Geometry check sheet. Reference: drawing and pictorial views, mm from the part's lowest x, y, z. A direction names the side the tool comes from. Round coordinates to 2 decimals unless told otherwise and drop trailing zeros. Loops run counter-clockwise (first coordinate to the right, second up) from the corner with the lowest first, then second, coordinate; pieces in that order, holes last. Notation, with made-up numbers: (-22.75, 59) - (19.25, 59) arc R22 cw to (19.25, 85) - close; hole circle Ø3 at (-9.75, -12.5). An arc over 180 degrees is marked (long way). Return JSON: item names as keys, results as strings.
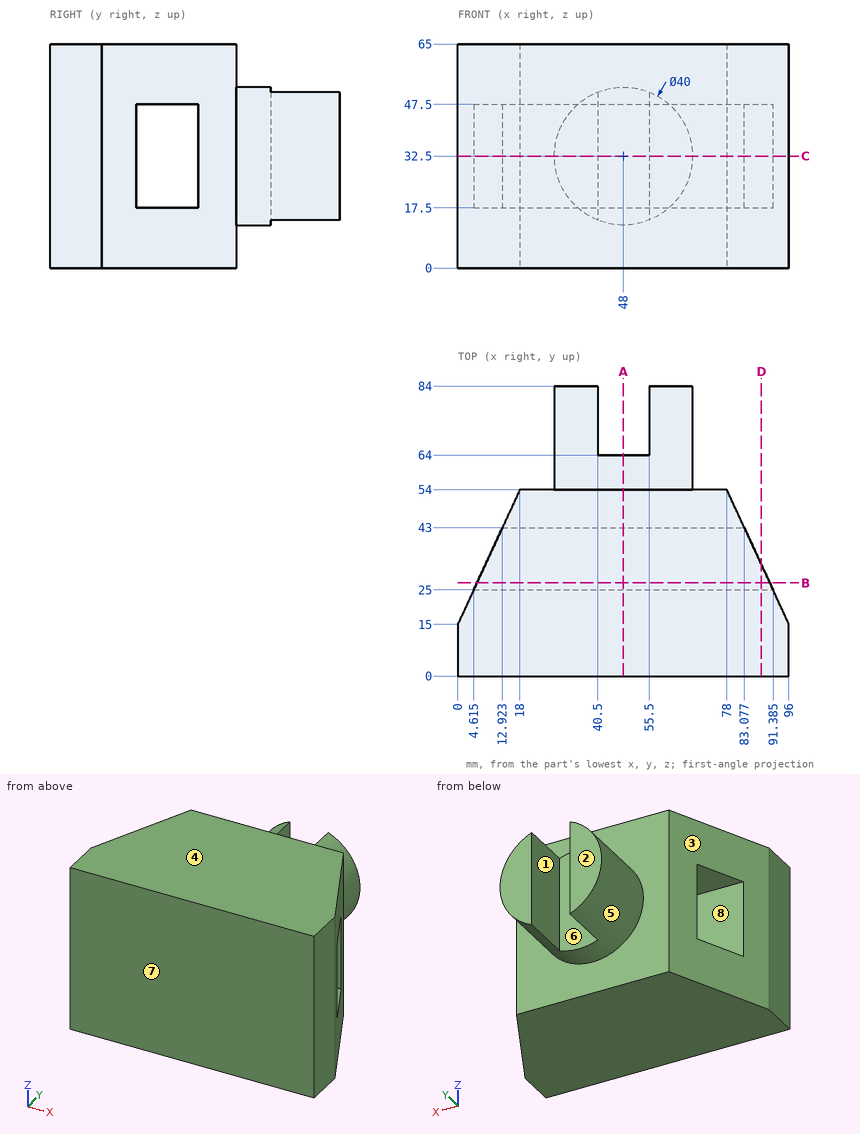
Q1. Scan lines: probe 1 along Y at (x, z) = (64, 47); probe 2 along Z at (x, y) = (34, 31); probe 3 along Y at (x, z) = (47.5, 18.5). Record each from-to range of solid material in increasing order. Write a range as [from, to].
Answer key:
{"probe 1": "y = [0, 25], [43, 54]", "probe 2": "z = [0, 17.5], [47.5, 65]", "probe 3": "y = [0, 25], [43, 64]"}
Q2. Sectioned sample at A-A (x = 48). Enter the section's corners in (y, z), plus the area to 3 significant figures.
Answer key:
{"outline": "(0, 0) - (54, 0) - (54, 12.5) - (64, 12.5) - (64, 52.5) - (54, 52.5) - (54, 65) - (0, 65) - close; hole (25, 17.5) - (43, 17.5) - (43, 47.5) - (25, 47.5) - close", "area": "3,370 mm²"}
Q3. Sectioned sample at B-B (y = 27). Enter the section's corners in (x, z).
Answer key:
{"outline": "(5.54, 0) - (90.46, 0) - (90.46, 17.5) - (5.54, 17.5) - close; (5.54, 47.5) - (90.46, 47.5) - (90.46, 65) - (5.54, 65) - close"}
Q4. Draft check along X on the marked faces 1, 2 and 3. Enter one of: released by +X, released by -X, zero draft, split by the parting line, or undercut.
Answer key:
{"face 1": "undercut", "face 2": "zero draft", "face 3": "released by -X"}
Q5. Depth check by flat-ended pin: P1, Ø12, axis at y = 62, z = 40, coming from the -X side; P2, Ø6, axis at y = 78.5, z = 36, coming from the -X side; P3, Ø22, axis at y = 76.5, z = 35, coming from the +X side. Enter the tip coordinate at first touch or a pass-through.
Answer key:
{"P1": "stops at x = 28.06", "P2": "stops at x = 28.01", "P3": "stops at x = 68"}
Q6. Tool access check on the marked faces 4, 5, 6, 7 and 8. Record the directions out of +Z, -Z, +X, -X, +Y, -Y that give a thin tool (end or side, any length) a straight path to the whole face; none if there is none.
Answer key:
{"face 4": "+Z, +X, -X, +Y, -Y", "face 5": "+Y", "face 6": "+Z, -Z, +Y", "face 7": "+Z, -Z, +X, -X, -Y", "face 8": "+X, -X"}
Q7. Sectioned sample at D-D (x = 88). Enter the section's corners in (y, z), plus the area to 3 significant figures.
Answer key:
{"outline": "(0, 0) - (32.33, 0) - (32.33, 17.5) - (25, 17.5) - (25, 47.5) - (32.33, 47.5) - (32.33, 65) - (0, 65) - close", "area": "1,880 mm²"}
Q8. Sectioned sample at C-C (z = 32.5). Enter the section's corners in (x, y) (1 decimal).
Answer key:
{"outline": "(0, 0) - (96, 0) - (96, 15) - (91.4, 25) - (4.6, 25) - (0, 15) - close; (12.9, 43) - (83.1, 43) - (78, 54) - (68, 54) - (68, 84) - (55.5, 84) - (55.5, 64) - (40.5, 64) - (40.5, 84) - (28, 84) - (28, 54) - (18, 54) - close"}
